Autodesk Inventor part; units mm, degrees
ref_plane "YZ Plane" through (0, 0, 0) normal (1, 0, 0) x (0, 1, 0)
ref_plane "XZ Plane" through (0, 0, 0) normal (0, 1, 0) x (-1, 0, 0)
ref_plane "XY Plane" through (0, 0, 0) normal (0, 0, 1) x (1, 0, 0)
sketch "Sketch1" plane through (0, 0, 0) normal (0, 0, 1) x (1, 0, 0)
  line L0 (0, 0) -> (-13.377, 0)
  line L1 (0, 0) -> (0, 26.67)
  line L2 (0, 26.67) -> (26.67, 0)
  line L3 (26.67, 0) -> (0, 0)
  dimension "d0" = 26.67
extrude "Extrusion1" add sketch "Sketch1" along normal mid plane 5.842
sketch "Sketch3" plane through (0, 0, 0) normal (0, 0, 1) x (1, 0, 0)
  line L0 (0, 26.67) -> (26.67, 0)
  line L1 (0, 0) -> (0, 26.67)
  line L2 (26.67, 0) -> (0, 0)
  line L3 (1.524, 25.146) -> (1.524, 1.524)
  line L4 (1.524, 1.524) -> (25.146, 1.524)
  line L5 (1.524, 25.146) -> (25.146, 1.524)
  dimension "d3" = 1.524
  dimension "d4" = 1.524
extrude "Extrusion2" cut sketch "Sketch3" against normal mid plane 2.032 contours L0 L4 L3
fillet "Fillet1" radius 1.524 3 edges at (0, 26.67, 0) (0, 0, 0) (26.67, 0, 0)
fillet "Fillet2" radius 1.016 6 edges at (0.4464, 0.4464, 2.921) (12.2574, 0, 2.921) (24.3987, 0.9408, 2.921) (13.335, 13.335, 2.921) (0.9408, 24.3987, 2.921) (0, 12.2574, 2.921)
fillet "Fillet3" radius 1.016 6 edges at (0.9408, 24.3987, -2.921) (13.335, 13.335, -2.921) (24.3987, 0.9408, -2.921) (12.2574, 0, -2.921) (0.4464, 0.4464, -2.921) (0, 12.2574, -2.921)
equation "\"d0\" = edgeSize"
equation "\"d1\" = partThickness"
equation "\"d3\" = edgeThickness"
equation "\"d4\" = edgeThickness"
equation "\"d5\" = mirrorThickness"
equation "\"d7\" = filetForCorners"
equation "\"d8\" = filetForFlat"
equation "\"d9\" = filetForFlat"
equation "\"edgeSize\" = 26.67"
equation "\"wallThickness\" = 1.905"
equation "\"mirrorThickness\" = 2.032"
equation "\"partThickness\" = mirrorThickness + 2 * wallThickness"
equation "\"edgeThickness\" = 1.524"
equation "\"filetForCorners\" = 1.524"
equation "\"filetForFlat\" = 1.016"
properties part number "Mirror Corner"
Geometry: final body of the model. Coordinates: model frame, mm. A direction names the side the tool comes from. Round coordinates to 2 decimals unless told otherwise and drop trailing zeros. Order: outer loops, then holes, each group sorted by start corner. A loop starts at its lowest first (then second) coordinate and runs counter-clockwise, first axis right, second up. Notation, with made-up numbers: (-10.5, 30) -> (35.5, 30) arc R15 cw to (35.5, 48) -> close; hole circle Ø3 at (0.25, 11.5). An arc over 180 degrees is marked (long way). Use CSV: the item, a comma, the result in double quotes. Start each with the question number.
1) Section A-A (z = 0.6). Return the cut outline in (x, y).
2) Material intervals for line 1 along Z through (x, y) = (18, 1.75); line 2 along X through (y, z) = (8.25, 0.75), sorted ascending. Write a range as from..to.
3) Set-up query: faces 1 (the face through (10, 11, -1.016)), 2 (the face through (12.107, 0.29, 2.615)). Return all of +Z, -Z, +X, -X, +Y, -Y with unobstructed straight access to the full face (end or side cutting, diameter ignored); none if empty.
4) Draft query along Z for faces 3 (the face through (0, 12, 0)), 4 (the face through (0.29, 12.408, 2.615)), 5 (the face through (12.98, 13.28, -2.615)), 6 (the face through (1.524, 13, 0)). Return one class per face: +Z half, -Z half, draft (parallel to the pull), parting line (faces both ways), or undercut.
5) First-contact query: pin 1 Ø1.6 at (y, z) = (15, 0.5) entering from +X; pin 2 Ø1.5 at (x, y) = (10.5, 15) entering from +Z; pin 3 Ø1.5 at (x, z) = (3.5, 0.5) entering from +Y. Flat tips, straight axial feed; report the tip coordinate or a pass-through.
Returned:
1,outline,"(0, 1.52) arc R1.52 ccw to (1.52, 0) -> (22.99, 0) arc R1.52 ccw to (24.51, 1.52) -> (1.52, 1.52) -> (1.52, 24.51) arc R1.52 ccw to (0, 22.99) -> close"
2,line 1,"z = -2.92..-1.02, 1.02..2.92"
2,line 2,"x = 0..1.52"
3,face 1,"+X, +Y"
3,face 2,"+Z, +X, -X, -Y"
4,face 3,"draft"
4,face 4,"+Z half"
4,face 5,"-Z half"
4,face 6,"undercut"
5,pin 1,"stops at x = 12.28"
5,pin 2,"stops at z = 2.92"
5,pin 3,"stops at y = 23.71"
